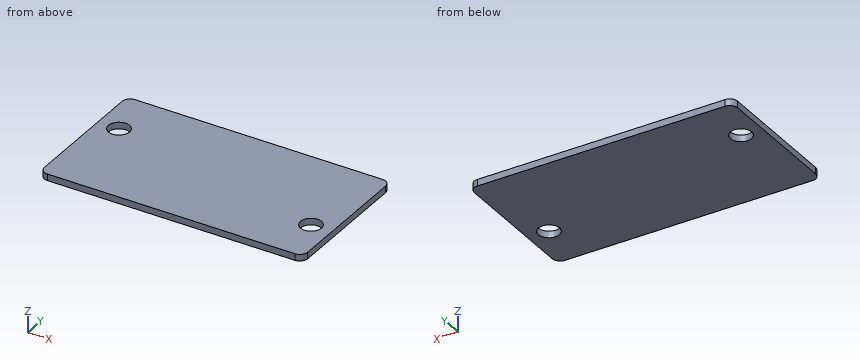
```python
from build123d import *

# Parameters (mm, degrees)
F0_W     = 1000
F0_H     = 340
F0_R     = 40
F1_DEPTH = 25


with BuildPart() as f1:
    # F0 (on Top) → F1 (new body)
    with BuildSketch(Plane.XY):
        with BuildLine():
            ThreePointArc((500, 240), (491.213203, 261.213203), (470, 270))
            Line((470, 270), (-470, 270))
            ThreePointArc((-470, 270), (-491.213203, 261.213203), (-500, 240))
            Line((-500, 240), (-500, 170))
            Line((-500, 170), (500, 170))
            Line((500, 170), (500, 240))
        make_face()
        with BuildLine():
            Line((500, -240), (500, -170))
            Line((500, -170), (-500, -170))
            Line((-500, -170), (-500, -240))
            ThreePointArc((-500, -240), (-491.213203, -261.213203), (-470, -270))
            Line((-470, -270), (470, -270))
            ThreePointArc((470, -270), (491.213203, -261.213203), (500, -240))
        make_face()
        Rectangle(F0_W, F0_H)
        with Locations((420, -90)):
            Circle(F0_R, mode=Mode.SUBTRACT)
        with Locations((-420, 90)):
            Circle(F0_R, mode=Mode.SUBTRACT)
    extrude(amount=F1_DEPTH)


solid = f1.part
```
Here's how the part is built. I have some questions about the finished solid (model axes, mm). Coordinates: 2 decimals unless noted, no trailing zeros. Write each loop counter-clockwise with the first axis right and the second up, starting at its lowest first coordinate (ties: lowest second). Pieces come first, ordered by that corner, then holes. Notation, with made-up numbers: (61, 51.25) - (69, 51.25) arc R27 ccw to (69, 76.25) - close; hole circle Ø10 at (-18, 73). An arc over 180 degrees is marked (long way). One line per item, written item: value.
1) Suppose I cut it at A-A on x = 420. Write out the boundary of the cut face in (y, z).
Model answer:
outline: (-270, 0) - (-130, 0) - (-130, 25) - (-270, 25) - close; (-50, 0) - (270, 0) - (270, 25) - (-50, 25) - close
2) I need wall thicknesses on line 1 along Y through (x, z) = (-420, 7.5); line 2 along Y through (x, z) = (420, 13); line 3 along X through (y, z) = (-59, 2.5). Which ranges of each line are inside material? Lowest first, please.
Model answer:
line 1: y = -270 to 50, 130 to 270
line 2: y = -270 to -130, -50 to 270
line 3: x = -500 to 394.72, 445.28 to 500
3) Suppose I cut it at B-B on y = 90. Write out the boundary of the cut face in (x, z).
Model answer:
outline: (-500, 0) - (-460, 0) - (-460, 25) - (-500, 25) - close; (-380, 0) - (500, 0) - (500, 25) - (-380, 25) - close
4) Suppose I cut it at C-C on z = 9.75. Write out the boundary of the cut face in (x, y).
Model answer:
outline: (-500, -240) arc R30 ccw to (-470, -270) - (470, -270) arc R30 ccw to (500, -240) - (500, 240) arc R30 ccw to (470, 270) - (-470, 270) arc R30 ccw to (-500, 240) - close; hole circle Ø80 at (-420, 90); hole circle Ø80 at (420, -90)
5) I'm going to push a flat-ended pin straight in: P1, Ø6, axis at x = -38.5, y = -103, coming from the -Z side. Where does the tip first touch, or does it pass through?
Model answer:
P1: stops at z = 0
